from build123d import *

# Parameters (mm, degrees)
F1_R     = 2.75
F1_R_2   = 1.7
F2_DEPTH = 3


with BuildPart() as f2:
    # F1 (on Top) → F2 (new body)
    with BuildSketch(Plane.XY):
        with BuildLine():
            Line((0, 0), (7, 0))
            Line((7, 0), (48.083883, 40.941477))
            Line((48.083883, 40.941477), (41, 48.05))
            Line((41, 48.05), (35, 48.05))
            ThreePointArc((35, 48.05), (27.928932, 50.978932), (25, 58.05))
            Line((25, 58.05), (25, 65.882149))
            ThreePointArc((25, 65.882149), (23.535534, 69.417683), (20, 70.882149))
            Line((20, 70.882149), (0, 70.882149))
            Line((0, 70.882149), (-20, 70.882149))
            ThreePointArc((-20, 70.882149), (-23.535534, 69.417683), (-25, 65.882149))
            Line((-25, 65.882149), (-25, 58.05))
            ThreePointArc((-25, 58.05), (-27.928932, 50.978932), (-35, 48.05))
            Line((-35, 48.05), (-41, 48.05))
            Line((-41, 48.05), (-48.083883, 40.941477))
            Line((-48.083883, 40.941477), (-7, 0))
            Line((-7, 0), (0, 0))
        make_face()
        with Locations((-7, 7)):
            Circle(F1_R, mode=Mode.SUBTRACT)
        with Locations((7, 7)):
            Circle(F1_R, mode=Mode.SUBTRACT)
        with BuildLine():
            Line((6.144092, 14.5), (0, 14.5))
            Line((0, 14.5), (-6.144092, 14.5))
            ThreePointArc((-6.144092, 14.5), (-7.289736, 14.727366), (-8.261726, 15.375))
            Line((-8.261726, 15.375), (-25.87277, 32.925))
            ThreePointArc((-25.87277, 32.925), (-26.52777, 36.195644), (-23.755136, 38.05))
            Line((-23.755136, 38.05), (0, 38.05))
            Line((0, 38.05), (23.755136, 38.05))
            ThreePointArc((23.755136, 38.05), (26.52777, 36.195644), (25.87277, 32.925))
            Line((25.87277, 32.925), (8.261726, 15.375))
            ThreePointArc((8.261726, 15.375), (7.289736, 14.727366), (6.144092, 14.5))
        make_face(mode=Mode.SUBTRACT)
        with Locations((-41, 40.882149)):
            Circle(F1_R, mode=Mode.SUBTRACT)
        with Locations((-21, 52.732149)):
            Circle(F1_R_2, mode=Mode.SUBTRACT)
        with Locations((-6, 52.732149)):
            Circle(F1_R_2, mode=Mode.SUBTRACT)
        with Locations((6, 52.732149)):
            Circle(F1_R_2, mode=Mode.SUBTRACT)
        with Locations((21, 52.732149)):
            Circle(F1_R_2, mode=Mode.SUBTRACT)
        with Locations((41, 40.882149)):
            Circle(F1_R, mode=Mode.SUBTRACT)
    extrude(amount=F2_DEPTH)


solid = f2.part
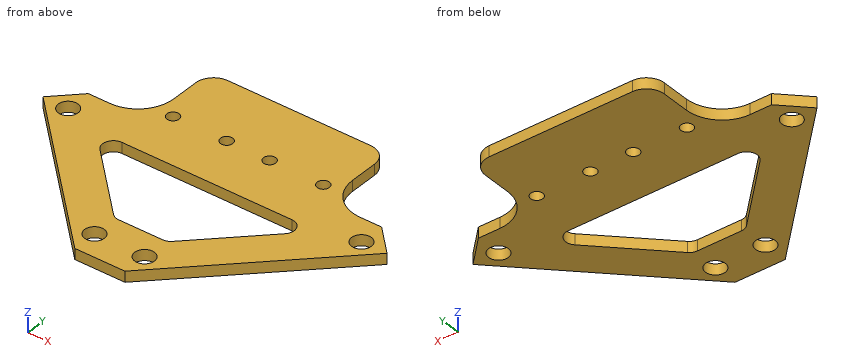
Can you work these out from the model? Positions are in its coordinate system, mm. Coordinates: 2 decimals unless noted, no trailing zeros. Write each loop counter-clockwise with the first axis right and the second up, starting at its lowest first coordinate (ties: lowest second). Pieces come first, ordered by that corner, then holes. Notation, with made-up numbers: (77.5, 10.25) -> (82.5, 10.25) arc R14 cw to (82.5, 35.25) -> close; hole circle Ø6 at (74, 30). An arc over 180 degrees is marked (long way). Write item = value, one per line.
(1) Imagine slicing it at B-B (x = 12.5). Please give me the cut outline in (y, z), and give its area (3 significant figures).
Verdict:
outline = (5.48, 0) -> (19.6, 0) -> (19.6, 3) -> (5.48, 3) -> close; (38.05, 0) -> (70.88, 0) -> (70.88, 3) -> (38.05, 3) -> close
area = 141 mm^2
(2) Imagine slicing it at C-C (z = 1.85). State how many separate pieces and enclosed holes the cut face has, and give its area (3 significant figures).
Verdict:
separate_pieces = 1
enclosed_holes = 9
area = 3,050 mm^2
(3) For pin 1 (6.5 mm diameter, centred on x = 7, y = 7, fed in from +Z); pin 2 (3.5 mm diameter, centred on x = -7, y = 7, fed in from -Z); pin 3 (1.5 mm diameter, centred on x = -37, z = 1, fed in from +Y); pin 4 (0.9 mm diameter, centred on y = 62.5, z = 2, fed in from -X), each with a flat end and sliding along its axis, tell me the tip position at first contact or that it passes through.
Verdict:
pin_1 = 3
pin_2 = through
pin_3 = 48.05
pin_4 = -25
(4) If I drill on probe 1 along Y at (x, z) = (2, 1); probe 2 along Y at (x, z) = (21, 0.8); probe 3 along Y at (x, z) = (-6, 1.9), over which ranges is the centre line in solid material (lowest first)?
Verdict:
probe_1 = 0 to 14.5, 38.05 to 70.88
probe_2 = 13.95 to 28.07, 38.05 to 51.03, 54.43 to 70.78
probe_3 = 0 to 4.44, 9.56 to 14.5, 38.05 to 51.03, 54.43 to 70.88
(5) Imagine slicing it at A-A (x = -21). Please give me the cut outline in (y, z), and give its area (3 significant figures).
Verdict:
outline = (13.95, 0) -> (28.07, 0) -> (28.07, 3) -> (13.95, 3) -> close; (38.05, 0) -> (51.03, 0) -> (51.03, 3) -> (38.05, 3) -> close; (54.43, 0) -> (70.78, 0) -> (70.78, 3) -> (54.43, 3) -> close
area = 130 mm^2
